Read the model definition and answer for the solid it produces. Units are mm, in the model's axes. Give positions to 0.01 mm unless a question says otherwise; leave off trailing zeros. Order: outer loops, then holes, each group sorted by start corner. A loop starts at its lowest first (then second) coordinate and runs counter-clockwise, first axis right, second up.
Item 1: A cutting plane is placed at C-C (z = -1.5). Write down the section's boundary in (x, y).
Item 2: A cutting plane is placed at A-A (x = 4.5). Write down the section's boundary in (y, z).
Item 3: A cutting plane is placed at B-B (y = -216). Write down the section's boundary in (x, z).
Item 4: Given pin 1 Ø2.5 at (y, z) = (-115.5, 0.5) entering from -X; pin 2 Ø5 at (y, z) = (-174, 1) entering from +X, each flat-ended and moving along its own axis, determine where each tip first touches the part or whether it passes through.
Item 5: Find the intervals of material crossed by line 1 along Z through (x, y) = (6.25, -166); line 2 along X through (y, z) = (-80, -4.5), in increasing order.
from build123d import *

# Parameters (mm, degrees)
F1_DEPTH = 254


with BuildPart() as f1:
    # F0 (on Front) → F1 (new body)
    with BuildSketch(Plane.XZ):
        Polygon((-1.524, 0), (0, 0), (0, 7.62), (-7.62, 7.62), (-7.62, 4.572), (-1.524, 4.572), align=None)
    extrude(amount=F1_DEPTH)

    # F2: F1 across face


with BuildPart() as f1_1:
    add(f1.part)
    add(f1.part.mirror(Plane(origin=(0, -127, 3.81), x_dir=(0, 1, 0), z_dir=(1, 0, 0))))

    # F3: F1 across face


with BuildPart() as f1_2:
    add(f1_1.part)
    add(f1_1.part.mirror(Plane(origin=(0, -127, 0), x_dir=(1, 0, 0), z_dir=(0, 0, -1))))


solid = f1_2.part
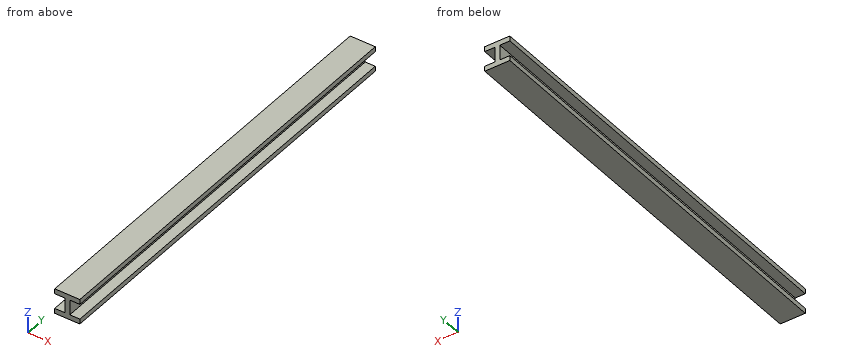
Response values:
1. outline: (-1.52, -254) - (1.52, -254) - (1.52, 0) - (-1.52, 0) - close
2. outline: (-254, -7.62) - (0, -7.62) - (0, -4.57) - (-254, -4.57) - close; (-254, 4.57) - (0, 4.57) - (0, 7.62) - (-254, 7.62) - close
3. outline: (-7.62, -7.62) - (7.62, -7.62) - (7.62, -4.57) - (1.52, -4.57) - (1.52, 4.57) - (7.62, 4.57) - (7.62, 7.62) - (-7.62, 7.62) - (-7.62, 4.57) - (-1.52, 4.57) - (-1.52, -4.57) - (-7.62, -4.57) - close
4. pin 1: stops at x = -1.52
4. pin 2: stops at x = 1.52
5. line 1: z = -7.62 to -4.57, 4.57 to 7.62
5. line 2: x = -1.52 to 1.52
